Verification items for the finished model (mm, model axes). A direction names the side the tool comes from. Round coordinates to 2 decimals unless told otherwise and drop trailing zeros. Write each loop counter-clockwise with the first axis right and the second up, starting at its lowest first coordinate (ties: lowest second). Pieces come first, ordered by that corner, then holes. Notation, with made-up numbers: (73.5, 42) -> (102.5, 42) arc R14 ccw to (102.5, 61) -> close; hole circle Ø3 at (67, 66). An arc over 180 degrees is marked (long way). Answer as a JSON object with one key per item and string values. Group by question number.
(1) Sectioned sample at D-D on x = 19. Record the cut outline in (y, z) (3 decimals), and give its area (3 significant figures).
(2) Set-up check for faces 1 (the face through (23.8, 34.8, 12)), 2 (the face through (3.175, 53, 13)): record each of +Z, -Z, +X, -X, +Y, -Y from which the full face is reachable in a straight line by a thin tool's end or side.
(3) Sectioned sample at A-A on z = 12.7. Record the cut outline in (x, y) (3 decimals).
(4) Sectioned sample at C-C on y = 38.1. Record the cut outline in (x, z) (3 decimals).
(5) Scan lines: L1, parallel to Y at x = 12.7, z = 24.1; L2, parallel to Y at x = 23.8, z = 12.7; L3, parallel to X at y = 50.5, z = 5.5 (3 decimals). Record each from-to range of solid material in increasing order. Write a range as from..to.
(6) Draft check along Z on faces 3 (the face through (13, 53, 25.4)), 4 (the face through (12.26, 73.12, 1.61)), 5 (the face through (22.225, 53, 13)). Enter one of: released by +Z, released by -Z, zero draft, split by the parting line, or undercut.
(7) Sectioned sample at B-B on x = 12.7. Count the separate pieces of the cut face and the enclosed holes in it, and give its area (3 significant figures).
Autodesk Inventor part; units mm, degrees
ref_plane "YZ Plane" through (0, 0, 0) normal (1, 0, 0) x (0, 1, 0)
ref_plane "XZ Plane" through (0, 0, 0) normal (0, 1, 0) x (-1, 0, 0)
ref_plane "XY Plane" through (0, 0, 0) normal (0, 0, 1) x (1, 0, 0)
sketch "Sketch1" plane through (0, 0, 0) normal (0, 1, 0) x (-1, 0, 0)
  line L0 (0, 0) -> (-25.4, 0)
  line L1 (-25.4, 0) -> (-25.4, 25.4)
  line L2 (-25.4, 25.4) -> (0, 25.4)
  line L3 (0, 25.4) -> (0, 0)
  line L4 (-22.225, 22.225) -> (-22.225, 3.175)
  line L5 (-22.225, 3.175) -> (-3.175, 3.175)
  line L6 (-3.175, 3.175) -> (-3.175, 22.225)
  line L7 (-3.175, 22.225) -> (-22.225, 22.225)
  dimension "d0" = 25.4
  dimension "d1" = 25.4
  dimension "d2" = 3.175
extrude "Extrusion1" add sketch "Sketch1" along normal blind 107.8738
sketch "Sketch2" plane through (0, 0, 25.4) normal (0, 0, 1) x (1, 0, 0)
  circle A0 centre (12.7, 95.1738) radius 3.3734
  line L0 (25.4, 0) -> (25.4, 107.8738)
  line L1 (0, 107.8738) -> (25.4, 107.8738)
  circle A1 centre (12.7, 69.7738) radius 3.3734
  circle A2 centre (12.7, 44.3738) radius 3.3734
  point P0 (0, 0)
  dimension "d5" = 6.7469
  dimension "d6" = 12.7
  dimension "d7" = 12.7
  dimension "d8" = 6.7469
  dimension "d9" = 12.7
  dimension "d10" = 25.4
  dimension "d11" = 6.7469
  dimension "d12" = 25.4
  dimension "d13" = 12.7
extrude "Extrusion2" cut sketch "Sketch2" against normal blind 25.4
sketch "Sketch3" plane through (0, 0, 0) normal (-1, 0, 0) x (0, 0, 1)
  circle A0 centre (12.7, 12.7) radius 3.3734
  circle A1 centre (12.7, 38.1) radius 3.3734
  line L0 (25.4, 0) -> (25.4, 107.8738)
  line L1 (25.4, 0) -> (0, 0)
  dimension "d16" = 6.7469
  dimension "d17" = 12.7
  dimension "d18" = 12.7
  dimension "d19" = 12.7
  dimension "d20" = 38.1
extrude "Extrusion3" cut sketch "Sketch3" against normal blind 25.4
properties part number "upright beam"
Computed values:
{
 "1": {"outline": "(0, 0) -> (107.874, 0) -> (107.874, 3.175) -> (0, 3.175) -> close; (0, 22.225) -> (107.874, 22.225) -> (107.874, 25.4) -> (0, 25.4) -> close", "area": "685 mm2"},
 "2": {"face 1": "+X, -X", "face 2": "+Y, -Y"},
 "3": {"outline": "(0, 0) -> (3.175, 0) -> (3.175, 9.327) -> (0, 9.327) -> close; (0, 16.073) -> (3.175, 16.073) -> (3.175, 34.727) -> (0, 34.727) -> close; (0, 41.473) -> (3.175, 41.473) -> (3.175, 107.874) -> (0, 107.874) -> close; (22.225, 0) -> (25.4, 0) -> (25.4, 9.327) -> (22.225, 9.327) -> close; (22.225, 16.073) -> (25.4, 16.073) -> (25.4, 34.727) -> (22.225, 34.727) -> close; (22.225, 41.473) -> (25.4, 41.473) -> (25.4, 107.874) -> (22.225, 107.874) -> close"},
 "4": {"outline": "(0, 0) -> (25.4, 0) -> (25.4, 9.327) -> (22.225, 9.327) -> (22.225, 3.175) -> (3.175, 3.175) -> (3.175, 9.327) -> (0, 9.327) -> close; (0, 16.073) -> (3.175, 16.073) -> (3.175, 22.225) -> (22.225, 22.225) -> (22.225, 16.073) -> (25.4, 16.073) -> (25.4, 25.4) -> (0, 25.4) -> close"},
 "5": {"L1": "0..41, 47.75..66.4, 73.15..91.8, 98.55..107.87", "L2": "0..9.33, 16.07..34.73, 41.47..107.87", "L3": "0..3.175, 22.225..25.4"},
 "6": {"face 3": "released by +Z", "face 4": "zero draft", "face 5": "undercut"},
 "7": {"separate pieces": "8", "enclosed holes": "0", "area": "556 mm2"}
}
